Source: CAD feature listing. Evaluate the final solid. Frame: model axes, mm. Round coordinates to 2 decimals unless told otherwise and drop trailing zeros. Loops run counter-clockwise (first coordinate to the right, second up) from the corner with the lowest first, then second, coordinate; pieces in that order, holes last. Notation, with made-up numbers: (83.25, 34.25) -> (92.25, 34.25) arc R15 cw to (92.25, 60.25) -> close; hole circle Ø9 at (1.25, -11.75). An arc over 180 degrees is marked (long way). Return JSON: item names as keys, results as strings. Group by question number.
```python
from build123d import *

# Parameters (mm, degrees)
SKETCH1_W                                = 250
SKETCH1_H                                = 150
BOSS_EXTRUDE1_DEPTH                      = 2
SKETCH2_R                                = 1.6
CUT_EXTRUDE1_DEPTH                       = 2
CUT_EXTRUDE2_DEPTH                       = 2
SKETCH10_R                               = 1.6
CUT_EXTRUDE7_DEPTH                       = 292.554454605
CUT_EXTRUDE8_DEPTH                       = 292.554454605
MIRROR5_AT_THE_SECOND_PLANE_COPY_1_DEPTH = 292.554454605
FILLET1_R                                = 10


with BuildPart() as part:
    # Sketch1 → Boss-Extrude1 (new body)
    with BuildSketch(Plane.XY):
        with Locations((125, 75)):
            Rectangle(SKETCH1_W, SKETCH1_H)
    extrude(amount=BOSS_EXTRUDE1_DEPTH)

    # Sketch2 → Cut-Extrude1 (cut)
    with BuildSketch(Plane.XY.offset(2)):
        with Locations((25, 140)):
            Circle(SKETCH2_R)
        with Locations((45, 140)):
            Circle(SKETCH2_R)
        with Locations((45, 115)):
            Circle(SKETCH2_R)
        with Locations((45, 90)):
            Circle(SKETCH2_R)
        with Locations((25, 115)):
            Circle(SKETCH2_R)
        with Locations((25, 90)):
            Circle(SKETCH2_R)
        with Locations((65, 140)):
            Circle(SKETCH2_R)
        with Locations((65, 115)):
            Circle(SKETCH2_R)
        with Locations((65, 90)):
            Circle(SKETCH2_R)
        with Locations((85, 140)):
            Circle(SKETCH2_R)
        with Locations((85, 115)):
            Circle(SKETCH2_R)
        with Locations((85, 90)):
            Circle(SKETCH2_R)
        with Locations(Location((165, 90, 0), (0, 0, 180))):
            Circle(SKETCH2_R)
        with Locations(Location((185, 90, 0), (0, 0, 180))):
            Circle(SKETCH2_R)
        with Locations(Location((205, 90, 0), (0, 0, 180))):
            Circle(SKETCH2_R)
        with Locations(Location((225, 90, 0), (0, 0, 180))):
            Circle(SKETCH2_R)
        with Locations(Location((225, 115, 0), (0, 0, 180))):
            Circle(SKETCH2_R)
        with Locations(Location((205, 115, 0), (0, 0, 180))):
            Circle(SKETCH2_R)
        with Locations(Location((185, 115, 0), (0, 0, 180))):
            Circle(SKETCH2_R)
        with Locations(Location((165, 115, 0), (0, 0, 180))):
            Circle(SKETCH2_R)
        with Locations(Location((165, 140, 0), (0, 0, 180))):
            Circle(SKETCH2_R)
        with Locations(Location((185, 140, 0), (0, 0, 180))):
            Circle(SKETCH2_R)
        with Locations(Location((205, 140, 0), (0, 0, 180))):
            Circle(SKETCH2_R)
        with Locations(Location((225, 140, 0), (0, 0, 180))):
            Circle(SKETCH2_R)
    cut_extrude1 = extrude(amount=-CUT_EXTRUDE1_DEPTH, mode=Mode.SUBTRACT)

    # Mirror1: Cut-Extrude1 across plane
    add(cut_extrude1.mirror(Plane(origin=(0, 75, 0), x_dir=(0, 0, 1), z_dir=(0, -1, 0))), mode=Mode.SUBTRACT)

    # Sketch5 → Cut-Extrude2 (cut)
    with BuildSketch(Plane.XY.offset(2)):
        with BuildLine():
            Line((23.4, 140), (23.4, 90))
            ThreePointArc((23.4, 90), (26.4, 87), (29.4, 90))
            Line((29.4, 90), (29.4, 140))
            ThreePointArc((29.4, 140), (26.4, 143), (23.4, 140))
        make_face()
        with BuildLine():
            Line((29.4, 10), (29.4, 60))
            ThreePointArc((29.4, 60), (26.4, 63), (23.4, 60))
            Line((23.4, 60), (23.4, 10))
            ThreePointArc((23.4, 10), (26.4, 7), (29.4, 10))
        make_face()
        with BuildLine():
            Line((226.6, 10), (226.6, 60))
            ThreePointArc((226.6, 60), (223.6, 63), (220.6, 60))
            Line((220.6, 60), (220.6, 10))
            ThreePointArc((220.6, 10), (223.6, 7), (226.6, 10))
        make_face()
        with BuildLine():
            Line((226.6, 140), (226.6, 90))
            ThreePointArc((226.6, 90), (223.6, 87), (220.6, 90))
            Line((220.6, 90), (220.6, 140))
            ThreePointArc((220.6, 140), (223.6, 143), (226.6, 140))
        make_face()
    extrude(amount=-CUT_EXTRUDE2_DEPTH, mode=Mode.SUBTRACT)

    # Sketch10 → Cut-Extrude7 (cut, through all)
    with BuildSketch(Plane.XY.offset(2)):
        with Locations((125, 140)):
            Circle(SKETCH10_R)
        with Locations((125, 35)):
            Circle(SKETCH10_R)
        with Locations((125, 60)):
            Circle(SKETCH10_R)
        with Locations((125, 88.292351152)):
            Circle(SKETCH10_R)
        with Locations((125, 113.292351152)):
            Circle(SKETCH10_R)
        with Locations((125, 10)):
            Circle(SKETCH10_R)
    extrude(amount=-CUT_EXTRUDE7_DEPTH, mode=Mode.SUBTRACT)

    # Sketch11 → Cut-Extrude8 (cut, through all)
    with BuildSketch(Plane.XY.offset(2)):
        with BuildLine():
            Line((99, 140), (99, 90))
            ThreePointArc((99, 90), (102, 87), (105, 90))
            Line((105, 90), (105, 140))
            ThreePointArc((105, 140), (102, 143), (99, 140))
        make_face()
    cut_extrude8 = extrude(amount=-CUT_EXTRUDE8_DEPTH, mode=Mode.SUBTRACT)

    # Mirror5: Cut-Extrude8 across plane
    add(cut_extrude8.mirror(Plane(origin=(0, 75, 0), x_dir=(0, 0, 1), z_dir=(0, -1, 0))), mode=Mode.SUBTRACT)

    # Mirror5 at the second plane: Cut-Extrude8 across plane
    add(cut_extrude8.mirror(Plane.ZY.offset(-125)), mode=Mode.SUBTRACT)

    # Mirror5 at the second plane copy 1 sketc → Mirror5 at the second plane copy 1 (cut, through all)
    with BuildSketch(Plane(origin=(250, 150, 2), x_dir=(-1, 0, 0), z_dir=(0, 0, 1))):
        with BuildLine():
            Line((99, 140), (99, 90))
            ThreePointArc((99, 90), (102, 87), (105, 90))
            Line((105, 90), (105, 140))
            ThreePointArc((105, 140), (102, 143), (99, 140))
        make_face()
    extrude(amount=-MIRROR5_AT_THE_SECOND_PLANE_COPY_1_DEPTH, mode=Mode.SUBTRACT)

    # Fillet1
    fillet1_edges = [part.edges().sort_by_distance(p)[0] for p in [
        (0, 150, 1),
        (250, 150, 1),
        (250, 0, 1),
        (0, 0, 1),
    ]]
    fillet(fillet1_edges, radius=FILLET1_R)


solid = part.part
```
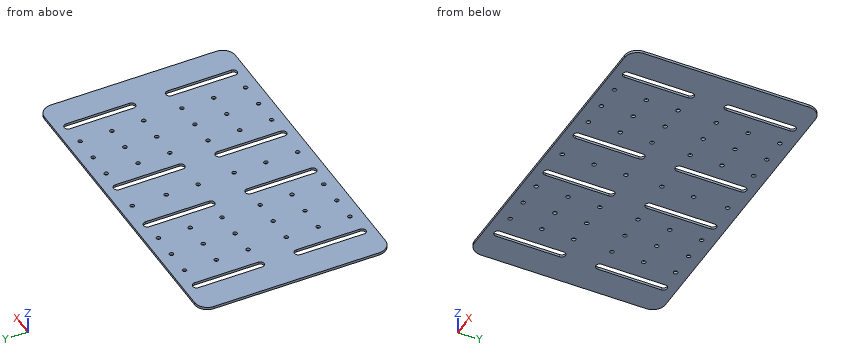
(1) Cut plane B-B (y = 133). Return loops of the section in (x, z), and give its area (3 significant figures).
(2) Cut plane C-C (z = 0.7). Count the separate pieces of the cut face and the enclosed holes in it, and give its area (3 significant figures).
(3) Ray query, line 1 (X direction, y = 98.5, z = 0.9); line 2 (Y direction, x = 28, z = 1.45). Return the intervals inside material, ascending.
(4) Cut plane A-A (x = 223.6). Return loops of the section in (y, z), and give its area (3 significant figures).
Answers follow:
{
 "1": {"outline": "(0, 0) -> (23.4, 0) -> (23.4, 2) -> (0, 2) -> close; (29.4, 0) -> (99, 0) -> (99, 2) -> (29.4, 2) -> close; (105, 0) -> (145, 0) -> (145, 2) -> (105, 2) -> close; (151, 0) -> (220.6, 0) -> (220.6, 2) -> (151, 2) -> close; (226.6, 0) -> (250, 0) -> (250, 2) -> (226.6, 2) -> close", "area": "452 mm^2"},
 "2": {"separate pieces": "1", "enclosed holes": "50", "area": "34,500 mm^2"},
 "3": {"line 1": "0 to 23.4, 29.4 to 99, 105 to 145, 151 to 220.6, 226.6 to 250", "line 2": "0 to 7.46, 62.54 to 87.46, 142.54 to 150"},
 "4": {"outline": "(0, 0) -> (7, 0) -> (7, 2) -> (0, 2) -> close; (63, 0) -> (87, 0) -> (87, 2) -> (63, 2) -> close; (143, 0) -> (150, 0) -> (150, 2) -> (143, 2) -> close", "area": "76.0 mm^2"}
}
